Source: CAD feature listing. Evaluate the final solid. Frame: model axes, mm. Face numbers are marked on the shaded views. Give positions to 0.01 mm unless a question says otherwise; leave off trailing zeros. Order: outer loops, then holes, each group sorted by start corner. A loop starts at its lowest first (then second) coordinate and runs counter-clockwise, first axis right, second up. Notation, with made-up numbers: (66, -13.5) - (101, -13.5) arc R33 ccw to (101, 16.5) - close; hole circle Ø1 at (59.25, -12). An arc over 180 degrees is marked (long way). Use CSV: the item, a comma, the result in double quotes.
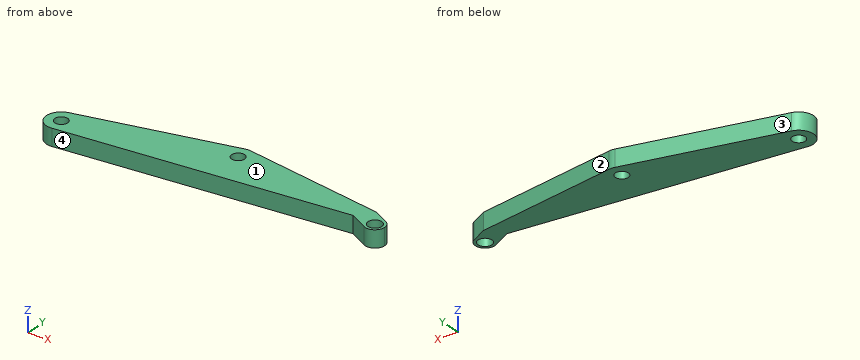
```python
from build123d import *

# Parameters (mm, degrees)
F0_R     = 1
F0_R_2   = 1.075
F1_DEPTH = 1.3


with BuildPart() as f1:
    # F0 (on Top) → F1 (new body)
    with BuildSketch(Plane.XY):
        with BuildLine():
            ThreePointArc((-1.724839, 5.20118), (-2.567642, 1.308568), (1.014279, 3.05))
            ThreePointArc((1.014279, 3.05), (0.477178, 4.49572), (-0.873565, 5.240085))
            ThreePointArc((-0.873565, 5.240085), (-1.301091, 5.26197), (-1.724839, 5.20118))
        make_face()
        with Locations((-1.2, 3.05)):
            Circle(F0_R, mode=Mode.SUBTRACT)
        with BuildLine():
            ThreePointArc((-0.873565, 5.240085), (0.477178, 4.49572), (1.014279, 3.05))
            ThreePointArc((1.014279, 3.05), (-2.567642, 1.308568), (-1.724839, 5.20118))
            Line((-1.724839, 5.20118), (-24.990567, -0.475129))
            ThreePointArc((-24.990567, -0.475129), (-23.041374, -0.897155), (-22.169366, -2.690773))
            ThreePointArc((-22.169366, -2.690773), (-22.75681, -4.218646), (-24.216514, -4.959423))
            Line((-24.216514, -4.959423), (19.374011, -0.473151))
            Line((19.374011, -0.473151), (22.209785, -1.955847))
            ThreePointArc((22.209785, -1.955847), (21.57553, 0.068436), (23.599812, 0.702691))
            Line((23.599812, 0.702691), (21.219947, 1.947013))
            Line((21.219947, 1.947013), (-0.873565, 5.240085))
        make_face()
        with BuildLine():
            ThreePointArc((-22.169366, -2.690773), (-23.041374, -0.897155), (-24.990567, -0.475129))
            ThreePointArc((-24.990567, -0.475129), (-26.697398, -3.078706), (-24.216514, -4.959423))
            ThreePointArc((-24.216514, -4.959423), (-22.75681, -4.218646), (-22.169366, -2.690773))
        make_face()
        with Locations((-24.45, -2.690773)):
            Circle(F0_R, mode=Mode.SUBTRACT)
        with BuildLine():
            ThreePointArc((24.404799, -0.626578), (24.187865, 0.150429), (23.599812, 0.702691))
            ThreePointArc((23.599812, 0.702691), (21.57553, 0.068436), (22.209785, -1.955847))
            ThreePointArc((22.209785, -1.955847), (23.681806, -1.909645), (24.404799, -0.626578))
        make_face()
        with Locations((22.904799, -0.626578)):
            Circle(F0_R_2, mode=Mode.SUBTRACT)
    extrude(amount=F1_DEPTH)

    # F2: F1 across plane


with BuildPart() as f1_1:
    add(f1.part)
    add(f1.part.mirror(Plane.XY))


solid = f1_1.part
```
Item 1: Section D-D on x = 14. Return the cut outline in (y, z), then the cut area to 3 significant figures.
Filled in:
outline,"(-1.03, -1.3) - (3.02, -1.3) - (3.02, 1.3) - (-1.03, 1.3) - close"
area,"10.5 mm2"
Item 2: Material intervals for line 1 (Y direction, x = -1.2, z = 0.55); line 2 (Y direction, x = -24.45, z = -0.75); line 3 (Y direction, x = 0, z = -0.9), sorted ascending. Write a range as from..to.
Filled in:
line 1,"y = -2.59..2.05, 4.05..5.26"
line 2,"y = -4.97..-3.69, -1.69..-0.34"
line 3,"y = -2.47..5.11"
Item 3: Mould query, pull axis X, two halves, no side actions, for the marked faces 1, 2, 3 and 4. Classes: released by +X, released by -X, zero draft, split by the parting line, or undercut.
Filled in:
face 1,"zero draft"
face 2,"released by +X"
face 3,"released by -X"
face 4,"undercut"
Item 4: Section A-A on y = 3.05. Return the cut outline in (x, z).
Filled in:
outline,"(-10.54, -1.3) - (-2.2, -1.3) - (-2.2, 1.3) - (-10.54, 1.3) - close; (-0.2, -1.3) - (13.82, -1.3) - (13.82, 1.3) - (-0.2, 1.3) - close"
Item 5: Section C-C on x = -6. Return the cut outline in (y, z), then the cut area to 3 significant figures.
Filled in:
outline,"(-3.08, -1.3) - (4.16, -1.3) - (4.16, 1.3) - (-3.08, 1.3) - close"
area,"18.8 mm2"
Item 6: Section B-B on z = -0.6. Return the cut outline in (x, y) (3 decimals), then the cut area to 3 significant figures.
Filled in:
outline,"(-24.991, -0.475) arc R2.281 ccw to (-24.217, -4.959) - (19.374, -0.473) - (22.21, -1.956) arc R1.5 ccw to (24.405, -0.627) arc R1.5 ccw to (23.6, 0.703) - (21.22, 1.947) - (-0.874, 5.24) arc R2.214 ccw to (-1.725, 5.201) - close; hole circle Ø2 at (-24.45, -2.691); hole circle Ø2 at (-1.2, 3.05); hole circle Ø2.15 at (22.905, -0.627)"
area,"268 mm2"
Item 7: First-contact query: pin 1 (1.8 mm diameter, centred on x = -24.45, y = -2.69, fed in from +Z). Flat tip, straight axial feed; report the tip coordinate or a pass-through.
Filled in:
pin 1,"passes through"
